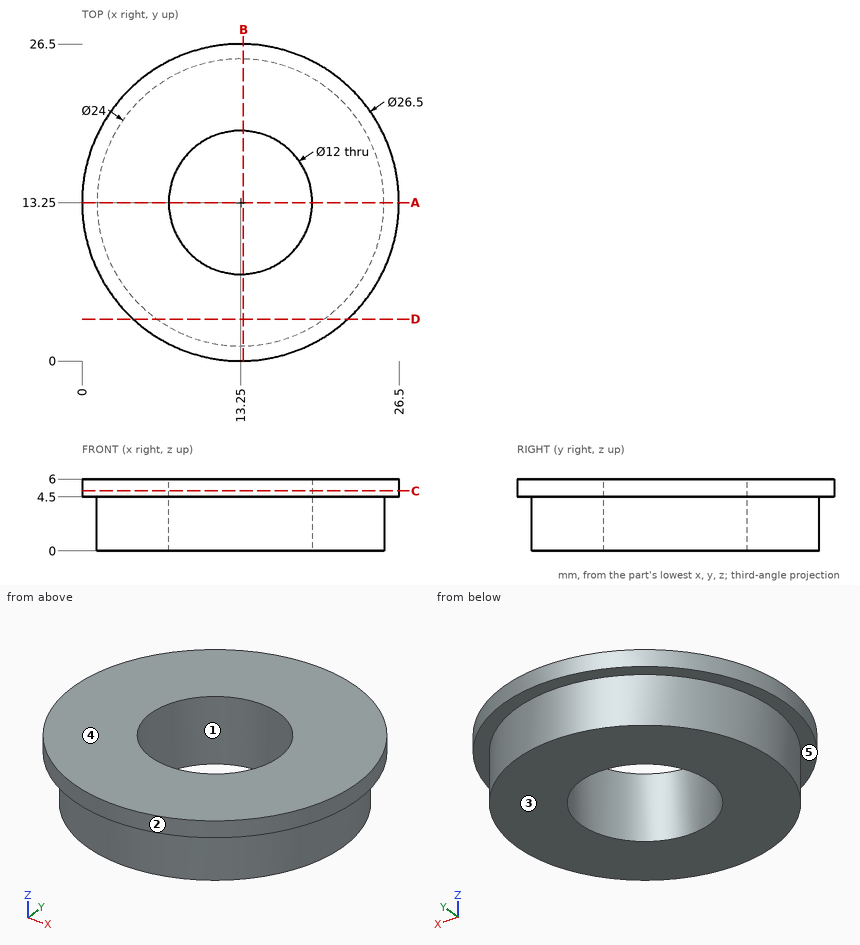
Study the drawing (mm; zero at the part's minimum x, y, z) and answer. A direction names the side the tool comes from. Round coordinates to 2 decimals unless told otherwise and drop trailing zeros. Loops run counter-clockwise (first coordinate to the right, second up) from the corner with the lowest first, then second, coordinate; pieces in that order, holes last. Notation, with made-up numbers: (31.25, 83) - (75.25, 83) arc R27 ccw to (75.25, 114) - close; hole circle Ø3 at (33, 54). An arc over 180 degrees is marked (long way). Use one line per item in the form item = value. Start each with the question number.
1. The part is cut by section A-A on y = 13.25. Determine the outline of the cut face in (x, z), then the cut area to 4 significant figures.
2. The part is cut by section C-C on z = 5. Determine the outline of the cut face in (x, y), then the cut area to 3 significant figures.
3. A tool of negligible diameter and unlimited length cuts with its end or side. For the marked faces 4 and 5, from which of +Z, -Z, +X, -X, +Y, -Y can it reach the whole face along a straight path? Write none if from no direction.
4. Given pin 1 Ø10 at (x, y) = (23, 4) entering from -Z; pin 2 Ø9.5 at (x, y) = (13.25, 13.25) entering from +Z; pin 3 Ø1.5 at (y, z) = (13, 3) entering from +X, each flat-ended and moving along its own axis, determine where each tip first touches the part or whether it passes through.
5. The part is cut by section D-D on y = 3.5. Determine the outline of the cut face in (x, z), then the cut area to 3 significant figures.
6. The part is cut by section B-B on x = 13.5. Determine the outline of the cut face in (y, z), then the cut area to 3 significant figures.
7. Consider line 1 (Y direction, x = 13.25, z = 4.65); line 2 (Y direction, x = 13.25, z = 4.1); line 3 (Z direction, x = 25.25, y = 10.75). Determine where each line is inside the solid, lowest interval first. Write a range as [from, to].
8. For a pull along Y with two mould halves and no side action, classify the marked faces 1, 2 and 3 as pulls with the +Y half, pulls with the -Y half, needs draft (parallel to the pull), parting line crosses it, or undercut.
Geometry check:
q1.outline = (0, 4.5) - (1.25, 4.5) - (1.25, 0) - (7.25, 0) - (7.25, 6) - (0, 6) - close; (19.25, 0) - (25.25, 0) - (25.25, 4.5) - (26.5, 4.5) - (26.5, 6) - (19.25, 6) - close
q1.area = 75.75 mm^2
q2.outline = circle Ø26.5 at (13.25, 13.25); hole circle Ø12 at (13.25, 13.25)
q2.area = 438 mm^2
q3.face_4 = +Z, +X, -X, +Y, -Y
q3.face_5 = -Z
q4.pin_1 = 0
q4.pin_2 = through
q4.pin_3 = 25.25
q5.outline = (4.28, 4.5) - (6.25, 4.5) - (6.25, 0) - (20.25, 0) - (20.25, 4.5) - (22.22, 4.5) - (22.22, 6) - (4.28, 6) - close
q5.area = 89.9 mm^2
q6.outline = (0, 4.5) - (1.25, 4.5) - (1.25, 0) - (7.26, 0) - (7.26, 6) - (0, 6) - close; (19.24, 0) - (25.25, 0) - (25.25, 4.5) - (26.5, 4.5) - (26.5, 6) - (19.24, 6) - close
q6.area = 75.8 mm^2
q7.line_1 = [0, 7.25], [19.25, 26.5]
q7.line_2 = [1.25, 7.25], [19.25, 25.25]
q7.line_3 = [4.5, 6]
q8.face_1 = undercut
q8.face_2 = parting line crosses it
q8.face_3 = needs draft
